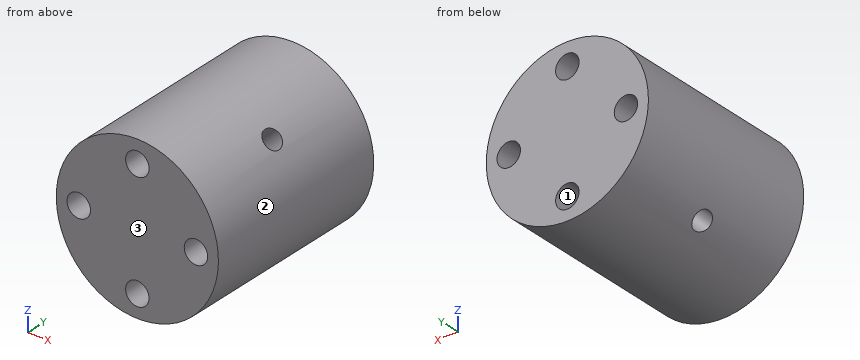
from build123d import *

# Parameters (mm, degrees)
SKETCH_1_R               = 10.375
EXTRUDE_1_DEPTH          = 25
SKETCH_2_R               = 1.5
CUT_EXTRUDE_1_DEPTH      = 29.98760511
CUT_EXTRUDE_2_DEPTH      = 29.98760511
CUT_EXTRUDE_2_DEPTH_BACK = 29.98760511
SKETCH_3_R               = 1.25


with BuildPart() as part:
    # Sketch 1 → Extrude 1 (new body)
    with BuildSketch(Plane(origin=(0, 0, 0), x_dir=(1, 0, 0), z_dir=(0, 1, 0))):
        with Locations(Location((0, 0, 0), (0, 0, 270))):
            Circle(SKETCH_1_R)
    extrude(amount=EXTRUDE_1_DEPTH)

    # Sketch 2 → Cut-Extrude 1 (cut, through all)
    with BuildSketch(Plane(origin=(0, 25, 0), x_dir=(1, 0, 0), z_dir=(0, 1, 0))):
        with Locations(Location((0, 7.5, 0), (0, 0, 270))):
            Circle(SKETCH_2_R)
        with Locations(Location((-7.5, 0, 0), (0, 0, 270))):
            Circle(SKETCH_2_R)
        with Locations(Location((7.5, 0, 0), (0, 0, 270))):
            Circle(SKETCH_2_R)
        with Locations(Location((0, -7.5, 0), (0, 0, 270))):
            Circle(SKETCH_2_R)
    extrude(amount=-CUT_EXTRUDE_1_DEPTH, mode=Mode.SUBTRACT)

    # Sketch 3 → Cut-Extrude 2 (cut, two sides: drawn at the far end of the back side and taken through both)
    with BuildSketch(Plane(origin=(0, 0, 0), x_dir=(0, 1, 0), z_dir=(0.7071067811865488, 0, 0.7071067811865464)).offset(-CUT_EXTRUDE_2_DEPTH_BACK)):
        with Locations(Location((12.5, 0, 0), (0, 0, 270))):
            Circle(SKETCH_3_R)
    extrude(amount=CUT_EXTRUDE_2_DEPTH + CUT_EXTRUDE_2_DEPTH_BACK, mode=Mode.SUBTRACT)


solid = part.part
Source: CAD feature listing. Evaluate the final solid. Frame: model axes, mm. Face numbers are marked on the shaded views. Round coordinates to 2 decimals unless told otherwise and drop trailing zeros. Write each loop counter-clockwise with the first axis right and the second up, starting at its lowest first coordinate (ties: lowest second). Pieces come first, ordered by that corner, then holes. Notation, with made-up numbers: M 3,34.25 L 29,34.25 A24 cw 29,48.25 Z; hole C -2.5,3.5 d1. An arc over 180 degrees is marked long. One line per item, written item: value. Start each with the question number.
Item 1: Mould query, pull axis Z, two halves, no side actions, for the marked faces 1, 2 and 3. Classes: pulls with the +Z half, pulls with the -Z half, needs draft (parallel to the pull), parting line crosses it, or undercut.
Item 2: Section query A-A (z = -8.5). Return the cut outline in (x, y), plus the area to 3 significant figures.
Item 3: Pin query (flat end, axial travel): pin 1 (1 mm diameter, centred on x = -7.5, y = 22.5, fed in from +Z); pin 2 (1.5 mm diameter, centred on x = -2.5, y = 8, fed in from +Z); pin 3 (10 mm diameter, centred on x = 6.5, y = 20.5, fed in from +Z). Return the tip coordinate at first contact, or that it passes through.
Item 4: Ray query, L1, parallel to X at y = 8.75, z = 0 (3 decimals); L2, parallel to X at y = 11, z = 1.25; L3, parallel to Y at x = -6.25, z = -5.5. Return the intervals inside material, ascending. Write a range as from..to.
Item 5: Section query B-B (y = 9.75). Return the cut outline in (x, z) (3 decimals).
Result set:
1. face 1: undercut
1. face 2: parting line crosses it
1. face 3: needs draft
2. outline: M -5.95,0 L -1.12,0 L -1.12,25 L -5.95,25 Z; M 1.12,0 L 5.95,0 L 5.95,25 L 1.12,25 Z
2. area: 242 mm²
3. pin 1: stops at z = 7.66
3. pin 2: stops at z = 10.23
3. pin 3: stops at z = 10.27
4. L1: x = -10.375..-9, -6..6, 9..10.375
4. L2: x = -10.3..-8.33, -6.67..6.67, 8.33..10.3
4. L3: y = 0..11.37, 13.63..25
5. outline: C 0,0 d20.75; hole C -7.5,0 d3; hole C 0,-7.5 d3; hole C 0,7.5 d3; hole C 7.5,0 d3
